Could you check a few things on this model? Use its own coordinates, in mm. A direction names the side the tool comes from. Round coordinates to 2 decimals unless told otherwise and drop trailing zeros. Order: outer loops, then holes, each group sorted by start corner. A loop starts at its lowest first (then second) coordinate and runs counter-clockwise, first axis right, second up. Notation, with made-up numbers: (49, -21) -> (92, -21) arc R28 cw to (92, -1) -> close; hole circle Ø4 at (-21.75, 88.25). An arc over 180 degrees is marked (long way). Put each result on its own line as item: value. Start each with the question number.
from build123d import *

# Parameters (mm, degrees)
CROQUIS1_W                 = 15
CROQUIS1_H                 = 45
CROQUIS1_W_2               = 7
CROQUIS1_H_2               = 14.8
SALIENTE_EXTRUIR1_DEPTH    = 5
CROQUIS2_W                 = 7
CROQUIS2_H                 = 14.8
SALIENTE_EXTRUIR4_DEPTH    = 18
CORTAR_EXTRUIR3_DEPTH      = 57.206405329
CORTAR_EXTRUIR3_DEPTH_BACK = 57.206405329


with BuildPart() as part:
    # Croquis1 → Saliente-Extruir1 (new body)
    # profile 1 of 4: a face of its own
    with BuildSketch(Plane.XY):
        with Locations((7.5, 22.5)):
            Rectangle(CROQUIS1_W, CROQUIS1_H)
        with Locations((9, 12.4)):
            Rectangle(CROQUIS1_W_2, CROQUIS1_H_2, mode=Mode.SUBTRACT)
    # profile 2 of 4: a face of its own
    with BuildSketch(Plane.XY):
        with Locations((22.5, 22.5)):
            Rectangle(CROQUIS1_W, CROQUIS1_H)
        with Locations((21, 12.4)):
            Rectangle(CROQUIS1_W_2, CROQUIS1_H_2, mode=Mode.SUBTRACT)
    # profile 3 of 4: a face of its own
    with BuildSketch(Plane.XY):
        with Locations((21, 12.4)):
            Rectangle(CROQUIS1_W_2, CROQUIS1_H_2)
    # profile 4 of 4: a face of its own
    with BuildSketch(Plane.XY):
        with Locations((9, 12.4)):
            Rectangle(CROQUIS1_W_2, CROQUIS1_H_2)
    extrude(amount=SALIENTE_EXTRUIR1_DEPTH)

    # Croquis2 → Saliente-Extruir4 (add)
    with BuildSketch(Plane.XY.offset(5)):
        with Locations((8.9, 12.4)):
            Rectangle(CROQUIS2_W, CROQUIS2_H)
        with Locations((21.1, 12.4)):
            Rectangle(CROQUIS2_W, CROQUIS2_H)
    extrude(amount=SALIENTE_EXTRUIR4_DEPTH)

    # Croquis4 → Cortar-Extruir3 (cut, two sides: drawn at the far end of the back side and taken through both)
    with BuildSketch(Plane.ZY.offset(-5.4).offset(-CORTAR_EXTRUIR3_DEPTH_BACK)):
        with BuildLine():
            Line((16, 14.74375), (16, 12.4))
            Line((16, 12.4), (18.34375, 12.4))
            ThreePointArc((18.34375, 12.4), (17.657281518, 14.057281518), (16, 14.74375))
        make_face()
        with BuildLine():
            Line((16, 10.05625), (16, 12.4))
            Line((16, 12.4), (13.65625, 12.4))
            ThreePointArc((13.65625, 12.4), (14.342718482, 10.742718482), (16, 10.05625))
        make_face()
        with BuildLine():
            Line((13.65625, 12.4), (16, 12.4))
            Line((16, 12.4), (16, 14.74375))
            ThreePointArc((16, 14.74375), (14.342718482, 14.057281518), (13.65625, 12.4))
        make_face()
        with BuildLine():
            Line((18.34375, 12.4), (16, 12.4))
            Line((16, 12.4), (16, 10.05625))
            ThreePointArc((16, 10.05625), (17.657281518, 10.742718482), (18.34375, 12.4))
        make_face()
        with BuildLine():
            ThreePointArc((16, 19.8), (20.97274021, 17.493132631), (23, 12.4))
            Line((23, 12.4), (23, 19.8))
            Line((23, 19.8), (16, 19.8))
        make_face()
        with BuildLine():
            Line((23, 5), (23, 12.4))
            ThreePointArc((23, 12.4), (20.97274021, 7.306867369), (16, 5))
            Line((16, 5), (23, 5))
        make_face()
    extrude(amount=CORTAR_EXTRUIR3_DEPTH + CORTAR_EXTRUIR3_DEPTH_BACK, mode=Mode.SUBTRACT)


solid = part.part
1. If we section it at B-B, the plane x = 9.5: Please give me the cut outline in (y, z), then the cut area to 3 significant figures.
2. Thinking about a two-plate mould opening in X: for faces 1 (the face through (15, 23, 0)), 2 (the face through (12.4, 12, 12)), 3 (the face through (24.6, 12, 12)), which applies, +X half, -X half, draft (parallel to the pull), parting line (faces both ways), or undercut?
3. For pin 1 Ø5 at (x, y) = (8.5, 6.5) entering from +Z; pin 2 Ø4.5 at (y, z) = (12, 11.5) entering from +X; pin 3 Ø3 at (x, y) = (12, 26.5) entering from -Z; pin 4 Ø3.5 at (x, z) = (22.5, 13) entering from +Y, each with a flat end and sliding along its axis, tell me the tip position at first contact or that it passes through.
4. I need wall thicknesses on L1, parallel to Z at x = 13.5, y = 32; L2, parallel to Y at x = 6, z = 9; L3, parallel to Y at x = 21.5, z = 17.5. Which ranges of each line are inside material? Lowest first, please.
5. If we section it at C-C, the plane y = 11.5: Please give me the cut outline in (x, z).
6. If we section it at A-A, the plane z = 10.5: Please give me the cut outline in (x, y).
7. Which directions (+Z, -Z, +X, -X, +Y, -Y) give clear straight access to the entire face, cutting with the end or side of a thin tool? Please do faces 4 (the face through (21, 5, 10)), 5 (the face through (21, 19.8, 10)), 6 (the face through (5.4, 12, 12)), 7 (the face through (17.6, 12, 12)).
8. If we section it at D-D, the plane z = 17.5: Please give me the cut outline in (x, y), then the cut area to 3 significant figures.
Results below:
1. outline: (0, 0) -> (45, 0) -> (45, 5) -> (19.8, 5) -> (19.8, 16) arc R7.41 ccw to (5, 16) -> (5, 5) -> (0, 5) -> close; hole circle Ø4.69 at (12.4, 16)
1. area: 451 mm2
2. face 1: draft
2. face 2: undercut
2. face 3: +X half
3. pin 1: z = 22.17
3. pin 2: x = 24.6
3. pin 3: z = 0
3. pin 4: y = 19.8
4. L1: 0 to 5
4. L2: 5 to 19.8
4. L3: 5.24 to 10.6, 14.2 to 19.56
5. outline: (0, 0) -> (30, 0) -> (30, 5) -> (24.6, 5) -> (24.6, 13.84) -> (17.6, 13.84) -> (17.6, 5) -> (12.4, 5) -> (12.4, 13.84) -> (5.4, 13.84) -> (5.4, 5) -> (0, 5) -> close; (5.4, 18.16) -> (12.4, 18.16) -> (12.4, 22.95) -> (5.4, 22.95) -> close; (17.6, 18.16) -> (24.6, 18.16) -> (24.6, 22.95) -> (17.6, 22.95) -> close
6. outline: (5.4, 5) -> (12.4, 5) -> (12.4, 19.8) -> (5.4, 19.8) -> close; (17.6, 5) -> (24.6, 5) -> (24.6, 19.8) -> (17.6, 19.8) -> close
7. face 4: +Z, +X, -X, -Y
7. face 5: +Z, +X, -X, +Y
7. face 6: +Z, -X, +Y, -Y
7. face 7: +Z, +Y, -Y
8. outline: (5.4, 5.24) -> (12.4, 5.24) -> (12.4, 10.6) -> (5.4, 10.6) -> close; (5.4, 14.2) -> (12.4, 14.2) -> (12.4, 19.56) -> (5.4, 19.56) -> close; (17.6, 5.24) -> (24.6, 5.24) -> (24.6, 10.6) -> (17.6, 10.6) -> close; (17.6, 14.2) -> (24.6, 14.2) -> (24.6, 19.56) -> (17.6, 19.56) -> close
8. area: 150 mm2
